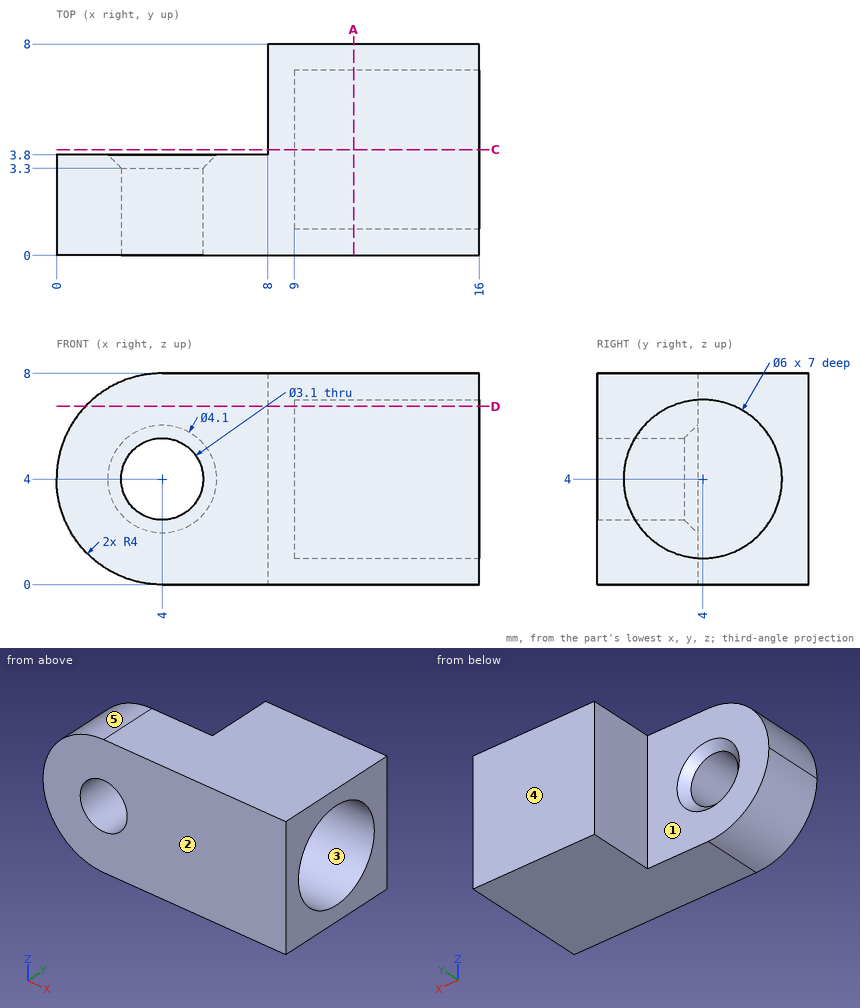
Here's the drawing with two shaded views (mm, measured from the low corner). I have some questions. A direction names the side the tool comes from. Give positions to 0.01 mm unless a question says otherwise; leave off trailing zeros. Write each loop counter-clockwise with the first axis right and the second up, starting at its lowest first coordinate (ties: lowest second). Pieces come first, ordered by that corner, then holes. Notation, with made-up numbers: (59, 76) - (85, 76) arc R22 ccw to (85, 94) - close; hole circle Ø9 at (-22.75, 64). An arc over 180 degrees is marked (long way). Write item = value, one per line. Start each with the question number.
1. Imagine slicing it at D-D (z = 6.75). Please give me the cut outline in (x, y) (3 decimals).
2. For pin 1 (1.5 mm diameter, centred on y = 1, z = 5, fed in from -X); pin 2 (4 mm diameter, centred on x = 2.5, y = 6.5, fed in from -Z); pin 3 (3 mm diameter, centred on x = 2, z = 5, fed in from +Y), each with a flat end and sliding along its axis, tell me the tip position at first contact or that it passes through.
3. On a 3-axis mill with a long thin cutter (end or side, diameter ignored), from which of +Z, -Z, +X, -X, +Y, -Y can I reach the whole of each face in a straight line? I mean the marked faces 1 and 2. Say none if no direction works.
4. Imagine slicing it at A-A (x = 11.25). Please give me the cut outline in (y, z).
5. Thinking about a two-plate mould opening in Y: for the marked faces 3, 4 and 5, which applies, released by +Y, released by -Y, zero draft, split by the parting line, or undercut?
6. Imagine slicing it at C-C (y = 4). Please give me the cut outline in (x, z), and give its area (3 significant figures).
7. Please list where these lines run through material, in increasing order: line 1 (Z direction, x = 13.75, y = 4); line 2 (Z direction, x = 4, y = 2.4); line 3 (Y direction, x = 5.5, z = 0.75).
Worked answers:
q1.outline = (1.095, 0) - (16, 0) - (16, 2.801) - (9, 2.801) - (9, 5.199) - (16, 5.199) - (16, 8) - (8, 8) - (8, 3.8) - (1.095, 3.8) - close
q2.pin_1 = 0.01
q2.pin_2 = through
q2.pin_3 = 3.8
q3.face_1 = +Z, -Z, -X, +Y
q3.face_2 = +Z, -Z, +X, -X, -Y
q4.outline = (0, 0) - (8, 0) - (8, 8) - (0, 8) - close; hole circle Ø6 at (4, 4)
q5.face_3 = undercut
q5.face_4 = released by +Y
q5.face_5 = zero draft
q6.outline = (8, 0) - (16, 0) - (16, 1) - (9, 1) - (9, 7) - (16, 7) - (16, 8) - (8, 8) - close
q6.area = 22.0 mm2
q7.line_1 = 0 to 1, 7 to 8
q7.line_2 = 0 to 2.45, 5.55 to 8
q7.line_3 = 0 to 3.8
